Check sheet for the modelled part. Datum: model origin and axes. Units: mm. Coordinates: 2 decimals unless noted, no trailing zeros. Loops run counter-clockwise (first coordinate to the right, second up) from the corner with the lowest first, then second, coordinate; pieces in that order, holes last.
from build123d import *

# Parameters (mm, degrees)
F1_DEPTH = 2
F2_D     = 5
F3_D     = 5


with BuildPart() as f1:
    # F0 (on Front) → F1 (new body)
    with BuildSketch(Plane.XZ):
        with BuildLine():
            ThreePointArc((0, 160), (-3.5355339059, 158.5355339059), (-5, 155))
            Line((-5, 155), (-5, -145))
            ThreePointArc((-5, -145), (-3.5355339059, -148.5355339059), (0, -150))
            ThreePointArc((0, -150), (3.5355339059, -148.5355339059), (5, -145))
            Line((5, -145), (5, 155))
            ThreePointArc((5, 155), (3.5355339059, 158.5355339059), (0, 160))
        make_face()
    extrude(amount=F1_DEPTH)

    # F2 (through all)
    with Locations(Plane(origin=(0, 0, 0), x_dir=(1, 0, 0), z_dir=(0, 1, 0))):
        with Locations((0, -155)):
            Hole(F2_D / 2)

    # F3 (through all)
    with Locations(Plane(origin=(0, 0, 0), x_dir=(1, 0, 0), z_dir=(0, 1, 0))):
        with Locations((0, 145)):
            Hole(F3_D / 2)


solid = f1.part
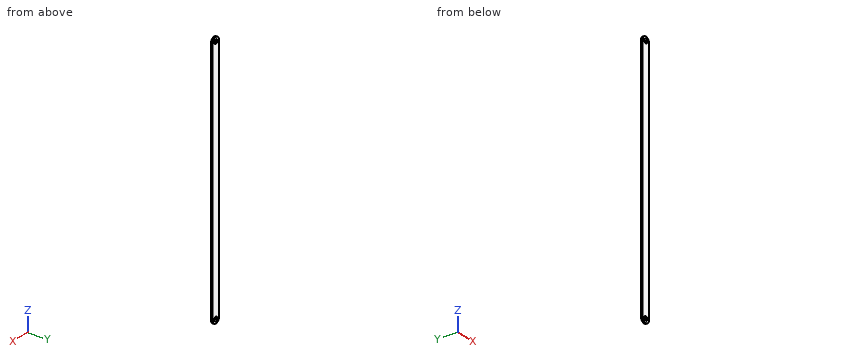
(1) Section check A-A, the plane y = -0.8. Enter the section's corners in (x, z), plus the area to 3 significant figures.
(2) Gauge pin test, flat end, axial feed: P1, Ø4, axis at x = 0, z = 155, coming from the +Y side. Record the tip position at first contact, or that the pin passes through.
(3) Scan lines: line 1 along Z through (x, y) = (-0.5, -0.85); line 2 along X through (y, z) = (-0.6, -145); line 3 along Z through (x, y) = (-2, -1.55). Record each from-to range of solid material in increasing order.
Determined:
1. outline: (-5, -145) arc R5 ccw to (5, -145) - (5, 155) arc R5 ccw to (-5, 155) - close; hole circle Ø5 at (0, -145); hole circle Ø5 at (0, 155)
1. area: 3,040 mm2
2. P1: passes through
3. line 1: z = -149.97 to -147.45, -142.55 to 152.55, 157.45 to 159.97
3. line 2: x = -5 to -2.5, 2.5 to 5
3. line 3: z = -149.58 to -146.5, -143.5 to 153.5, 156.5 to 159.58
